Geometry check sheet. Reference: the model listing, model coordinates, mm. A direction names the side the tool comes from. Coordinates: 2 decimals unless noted, no trailing zeros. Loops run counter-clockwise (first coordinate to the right, second up) from the corner with the lowest first, then second, coordinate; pieces in that order, holes last.
from build123d import *

# Parameters (mm, degrees)
SKETCH1_R           = 1.685173155
BOSS_EXTRUDE2_DEPTH = 2.54
FILLET1_R           = 1.27


with BuildPart() as part:
    # Sketch1 → Boss-Extrude2 (new body)
    with BuildSketch(Plane(origin=(0, 0, 0), x_dir=(1, 0, 0), z_dir=(0, 1, 0))):
        with BuildLine():
            Line((7.25, 42.9514), (-7.25, 42.9514))
            ThreePointArc((-7.25, 42.9514), (-7.603553391, 43.097846609), (-7.75, 43.4514))
            Line((-7.75, 43.4514), (-7.75, 45.9994))
            Line((-7.75, 45.9994), (-17.907, 45.9994))
            Line((-17.907, 45.9994), (-17.907, 54.8894))
            ThreePointArc((-17.907, 54.8894), (-18.278974388, 55.787425612), (-19.177, 56.1594))
            Line((-19.177, 56.1594), (-22.987, 56.1594))
            ThreePointArc((-22.987, 56.1594), (-23.885025612, 55.787425612), (-24.257, 54.8894))
            Line((-24.257, 54.8894), (-24.257, 45.9994))
            Line((-24.257, 45.9994), (-36.957, 45.9994))
            ThreePointArc((-36.957, 45.9994), (-38.753051224, 45.255451224), (-39.497, 43.4594))
            Line((-39.497, 43.4594), (-39.497, -43.4594))
            ThreePointArc((-39.497, -43.4594), (-38.753051224, -45.255451224), (-36.957, -45.9994))
            Line((-36.957, -45.9994), (-7.75, -45.9994))
            Line((-7.75, -45.9994), (-7.75, -43.4514))
            ThreePointArc((-7.75, -43.4514), (-7.603553391, -43.097846609), (-7.25, -42.9514))
            Line((-7.25, -42.9514), (7.25, -42.9514))
            ThreePointArc((7.25, -42.9514), (7.603553391, -43.097846609), (7.75, -43.4514))
            Line((7.75, -43.4514), (7.75, -45.9994))
            Line((7.75, -45.9994), (17.907, -45.9994))
            Line((17.907, -45.9994), (17.907, -54.8894))
            ThreePointArc((17.907, -54.8894), (18.278974388, -55.787425612), (19.177, -56.1594))
            Line((19.177, -56.1594), (22.987, -56.1594))
            ThreePointArc((22.987, -56.1594), (23.885025612, -55.787425612), (24.257, -54.8894))
            Line((24.257, -54.8894), (24.257, -45.9994))
            Line((24.257, -45.9994), (36.957, -45.9994))
            ThreePointArc((36.957, -45.9994), (38.753051224, -45.255451224), (39.497, -43.4594))
            Line((39.497, -43.4594), (39.497, 43.4594))
            ThreePointArc((39.497, 43.4594), (38.753051224, 45.255451224), (36.957, 45.9994))
            Line((36.957, 45.9994), (7.75, 45.9994))
            Line((7.75, 45.9994), (7.75, 43.4514))
            ThreePointArc((7.75, 43.4514), (7.603553391, 43.097846609), (7.25, 42.9514))
        make_face()
        with BuildLine():
            ThreePointArc((16.997, 41.4994), (17.582786438, 42.913613562), (18.997, 43.4994))
            Line((18.997, 43.4994), (34.997, 43.4994))
            ThreePointArc((34.997, 43.4994), (36.411213562, 42.913613562), (36.997, 41.4994))
            Line((36.997, 41.4994), (36.997, -41.4994))
            ThreePointArc((36.997, -41.4994), (36.411213562, -42.913613562), (34.997, -43.4994))
            Line((34.997, -43.4994), (18.997, -43.4994))
            ThreePointArc((18.997, -43.4994), (17.582786438, -42.913613562), (16.997, -41.4994))
            Line((16.997, -41.4994), (16.997, 41.4994))
        make_face(mode=Mode.SUBTRACT)
        with Locations(Location((-21.082, 52.3494, 0), (0, 0, 270))):
            Circle(SKETCH1_R, mode=Mode.SUBTRACT)
        with Locations(Location((21.082, -52.3494, 0), (0, 0, 270))):
            Circle(SKETCH1_R, mode=Mode.SUBTRACT)
    extrude(amount=BOSS_EXTRUDE2_DEPTH)

    # Fillet1
    fillet1_edges = [part.edges().sort_by_distance(p)[0] for p in [
        (-24.257, 1.27, -45.9994),
        (-17.907, 1.27, -45.9994),
        (24.257, 1.27, 45.9994),
        (17.907, 1.27, 45.9994),
    ]]
    fillet(fillet1_edges, radius=FILLET1_R)


solid = part.part
1) Section check B-B on x = 27.5. Record the cut outline in (y, z).
Data:
outline: (0, -46) - (2.54, -46) - (2.54, -43.5) - (0, -43.5) - close; (0, 43.5) - (2.54, 43.5) - (2.54, 46) - (0, 46) - close
2) Material ranges on probe 1 along X at (y, z) = (1.2, 0); probe 2 along Z at (x, y) = (23, 2.25); probe 3 along Z at (x, y) = (-21, 0.1), recorded low to high.
Data:
probe 1: x = -39.5 to 17, 37 to 39.5
probe 2: z = -46 to -43.5, 43.5 to 56.16
probe 3: z = -56.16 to -54.03, -50.67 to 46
3) Access from +Z, -Z, +X, -X, +Y, -Y to the whole of each face (thin tool, end or side, straight path). Record for faces 4 (the flat face through (-12, 1, -45.999)), 5 (the flat face through (17.907, 1, 51)), 6 (the flat face through (0, 1, -42.951)).
Data:
face 4: -Z, +X, +Y, -Y
face 5: +Z, -X, +Y, -Y
face 6: -Z, +Y, -Y
4) Section check D-D on y = 2.1. Count the separate pieces of the cut face and the enclosed holes in it, and give its area (3 significant figures).
Data:
separate pieces: 1
enclosed holes: 3
area: 5,540 mm2
5) Depth check by flat-ended pin: pin 1 (1.3 mm diameter, centred on y = 1, z = -50, fed in from +X); pin 2 (0.8 mm diameter, centred on y = 0.5, z = -51.5, fed in from -X); pin 3 (0.8 mm diameter, centred on x = -2.5, y = 1, fed in from -Z); pin 4 (3 mm diameter, centred on x = 21.08, z = 52.35, fed in from -Y). Enter the tip coordinate at first touch or a pass-through.
Data:
pin 1: stops at x = -17.91
pin 2: stops at x = -24.26
pin 3: stops at z = -42.95
pin 4: passes through
6) Section check C-C on x = -1. Record the cut outline in (y, z), and give its area (3 significant figures).
Data:
outline: (0, -42.95) - (2.54, -42.95) - (2.54, 42.95) - (0, 42.95) - close
area: 218 mm2
7) Section check A-A on z = -33. Record the cut outline in (x, y), and give its area (3 significant figures).
Data:
outline: (-39.5, 0) - (17, 0) - (17, 2.54) - (-39.5, 2.54) - close; (37, 0) - (39.5, 0) - (39.5, 2.54) - (37, 2.54) - close
area: 150 mm2
8) Mould release check, pull along X, two halves, no side actions. Record for faces 1 (the cylindrical face through (-38.73, 1.25, -45.28)), 2 (the flat face through (0, 1, 42.951)), 3 (the flat face through (-18, 2.54, -1)): +X half, -X half, draft (parallel to the pull), parting line (faces both ways), or undercut.
Data:
face 1: -X half
face 2: undercut
face 3: draft
